Print and shaded views of the part. All mm, measured from the part's lowest x, y and z. A direction names the side the tool comes from. Round coordinates to 2 decimals unless told otherwise and drop trailing zeros. Order: outer loops, then holes, each group sorted by start corner. A loop starts at its lowest first (then second) coordinate and runs counter-clockwise, first axis right, second up. Notation, with made-up numbers: (63, 78.25) - (74, 78.25) arc R32 cw to (74, 116.25) - close; hole circle Ø11 at (55, 66). An arc over 180 degrees is marked (long way). Write item = value, one per line.
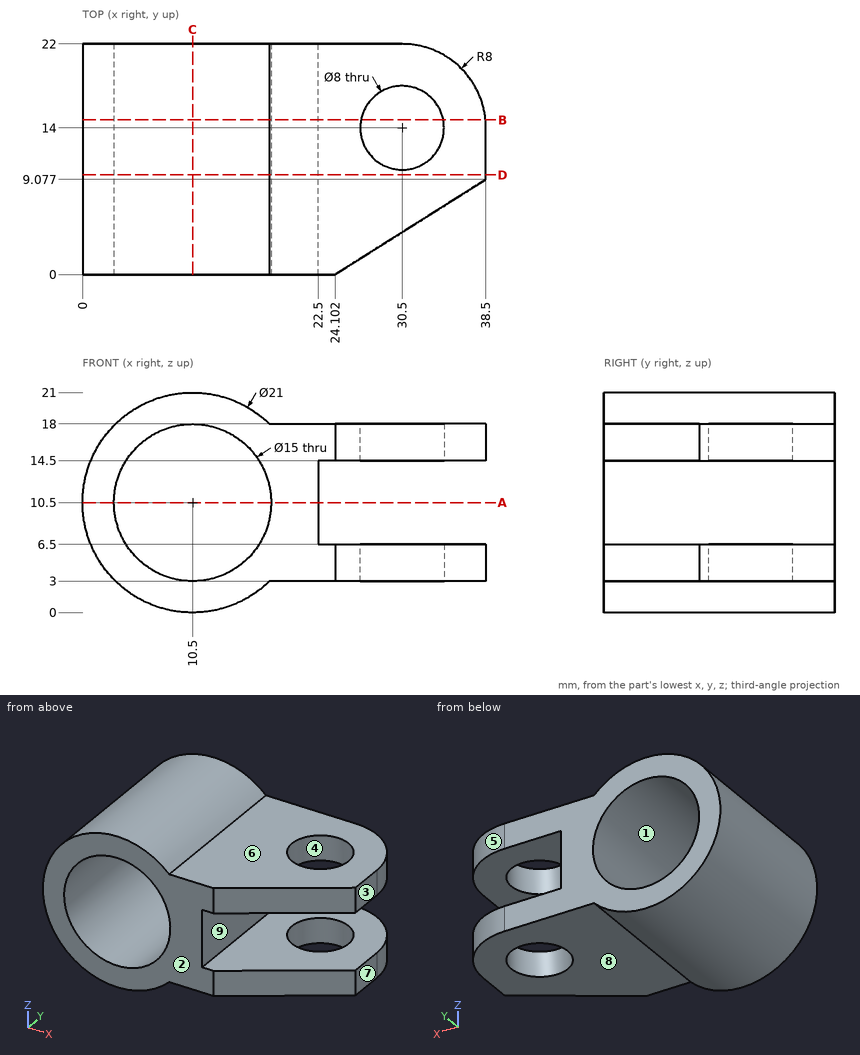
(1) Pull direction X, two halves, no side cores. Call the marked faces 1, 2, 3 and 4: released by +X, released by -X, zero draft, split by the parting line, or undercut.
Solved:
face_1 = undercut
face_2 = zero draft
face_3 = released by +X
face_4 = undercut
(2) Band-saw the part on D-D on y = 9.5. List the corners of the cut face in (x, z), plus the area to 3 significant figures.
Solved:
outline = (17.85, 3) - (38.5, 3) - (38.5, 6.5) - (22.5, 6.5) - (22.5, 14.5) - (38.5, 14.5) - (38.5, 18) - (17.85, 18) arc R10.5 ccw (long way) to start; hole circle Ø15 at (10.5, 10.5)
area = 319 mm²
(3) Probe line 1 along Z through (x, y) = (28, 21); line 2 along X through (y, z) = (14.75, 10.5); line 3 along Z through (x, y) = (5, 6.5) (1 decimal). List the from-to ranges inside material, lowest first.
Solved:
line_1 = 3 to 6.5, 14.5 to 18
line_2 = 0 to 3, 18 to 22.5
line_3 = 1.6 to 5.4, 15.6 to 19.4
(4) Tool access for the marked faces 5, 6, 7, 8 and 9: list every direction of +Z, -Z, +X, -X, +Y, -Y with a clear straight run to the whole face (end or side of a thin tool).
Solved:
face_5 = +Z, -Z, +X, +Y
face_6 = +Z, +X, +Y, -Y
face_7 = +Z, -Z, +X, +Y, -Y
face_8 = -Z, +X, +Y, -Y
face_9 = +X, +Y, -Y
(5) Drop flat-ended pins along their axis: pin 1 (1 mm diameter, centred on x = 27, y = 7, fed in from +Z); pin 2 (1.5 mm diameter, centred on y = 5, z = 14, fed in from +X); pin 3 (8 mm diameter, centred on x = 29.5, y = 6, fed in from -Z). Give the stop position or say it passes through.
Solved:
pin_1 = 18
pin_2 = 32.92
pin_3 = 3
(6) Band-saw the part on B-B on y = 14.75. List the corners of the cut face in (x, z) (1 decimal).
Solved:
outline = (17.8, 3) - (26.6, 3) - (26.6, 6.5) - (22.5, 6.5) - (22.5, 14.5) - (26.6, 14.5) - (26.6, 18) - (17.8, 18) arc R10.5 ccw (long way) to start; (34.4, 3) - (38.5, 3) - (38.5, 6.5) - (34.4, 6.5) - close; (34.4, 14.5) - (38.5, 14.5) - (38.5, 18) - (34.4, 18) - close; hole circle Ø15 at (10.5, 10.5)
(7) Band-saw the part on C-C on x = 10.5. List the corners of the cut face in (y, z), plus the area to 3 significant figures.
Solved:
outline = (0, 0) - (22, 0) - (22, 3) - (0, 3) - close; (0, 18) - (22, 18) - (22, 21) - (0, 21) - close
area = 132 mm²
(8) Band-saw the part on A-A on z = 10.5. List the corners of the cut face in (x, y).
Solved:
outline = (0, 0) - (3, 0) - (3, 22) - (0, 22) - close; (18, 0) - (22.5, 0) - (22.5, 22) - (18, 22) - close
